from build123d import *

# Parameters (mm, degrees)
CROQUIS4_R              = 11
SALIENTE_EXTRUIR2_DEPTH = 25
CROQUIS5_R              = 3
SALIENTE_EXTRUIR3_DEPTH = 1.5
CROQUIS6_R              = 1.5
SALIENTE_EXTRUIR4_DEPTH = 0.5
CROQUIS7_R              = 1
SALIENTE_EXTRUIR5_DEPTH = 6
REDONDEO1_R             = 1
CROQUIS10_R             = 9.905946753
SALIENTE_EXTRUIR6_DEPTH = 1
CORTAR_EXTRUIR1_START   = 1
CROQUIS8_R              = 1.25
CORTAR_EXTRUIR1_DEPTH   = 6


with BuildPart() as part:
    # Croquis4 → Saliente-Extruir2 (new body)
    with BuildSketch(Plane(origin=(0, 0, 0), x_dir=(0, 0, -1), z_dir=(1, 0, 0))):
        Circle(CROQUIS4_R)
    extrude(amount=SALIENTE_EXTRUIR2_DEPTH)

    # Croquis5 → Saliente-Extruir3 (add)
    with BuildSketch(Plane(origin=(25, 0, 0), x_dir=(0, 0, -1), z_dir=(1, 0, 0))):
        Circle(CROQUIS5_R)
    extrude(amount=SALIENTE_EXTRUIR3_DEPTH)

    # Croquis6 → Saliente-Extruir4 (add)
    with BuildSketch(Plane(origin=(26.5, 0, 0), x_dir=(0, 0, -1), z_dir=(1, 0, 0))):
        Circle(CROQUIS6_R)
    extrude(amount=SALIENTE_EXTRUIR4_DEPTH)

    # Croquis7 → Saliente-Extruir5 (add)
    with BuildSketch(Plane(origin=(27, 0, 0), x_dir=(0, 0, -1), z_dir=(1, 0, 0))):
        Circle(CROQUIS7_R)
    extrude(amount=SALIENTE_EXTRUIR5_DEPTH)

    # Redondeo1
    redondeo1_edges = [part.edges().sort_by_distance(p)[0] for p in [
        (33, 0, 1),
    ]]
    fillet(redondeo1_edges, radius=REDONDEO1_R)

    # Croquis10 → Saliente-Extruir6 (add)
    with BuildSketch(Plane(origin=(25, 0, 0), x_dir=(0, 0, -1), z_dir=(1, 0, 0))):
        Circle(CROQUIS10_R)
    extrude(amount=SALIENTE_EXTRUIR6_DEPTH)

    # Croquis9 → Cortar-Revolución2 (revolve, cut)
    with BuildSketch(Plane.XY, mode=Mode.PRIVATE) as cortar_revoluci_n2_sk:
        Polygon((3.71935431, 11), (0, 11), (0, 10), (2.798724642, 10), align=None)
    revolve(cortar_revoluci_n2_sk.sketch.rotate(Axis((0, 0, 0), (1, 0, 0)), 90), axis=Axis((0, 0, 0), (1, 0, 0)), mode=Mode.SUBTRACT)

    # Croquis8 → Cortar-Extruir1 (cut)
    with BuildSketch(Plane(origin=(25, 0, 0), x_dir=(0, 0, -1), z_dir=(1, 0, 0)).offset(CORTAR_EXTRUIR1_START)):
        with Locations((0, 6)):
            Circle(CROQUIS8_R)
        with Locations((5.196152423, 3)):
            Circle(CROQUIS8_R)
        with Locations((5.196152423, -3)):
            Circle(CROQUIS8_R)
        with Locations((0, -6)):
            Circle(CROQUIS8_R)
        with Locations((-5.196152423, -3)):
            Circle(CROQUIS8_R)
        with Locations((-5.196152423, 3)):
            Circle(CROQUIS8_R)
    extrude(amount=-CORTAR_EXTRUIR1_DEPTH, mode=Mode.SUBTRACT)


solid = part.part
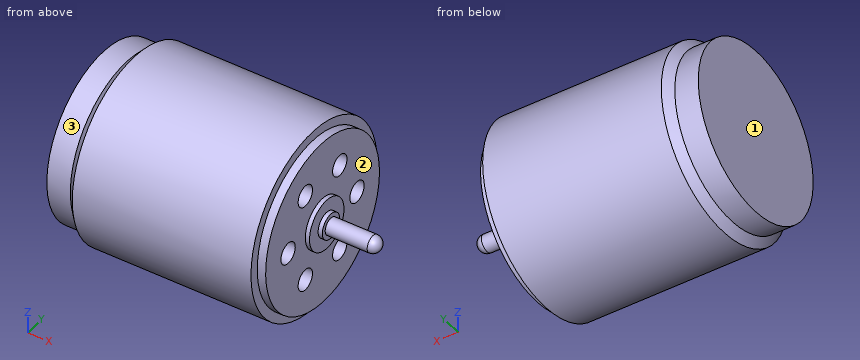
Verification items for the finished model (mm, model axes). Face numbers are marked on the shaded views. A direction names the side the tool comes from. Coordinates: 2 decimals unless noted, no trailing zeros. Write each loop counter-clockwise with the first axis right and the second up, starting at its lowest first coordinate (ties: lowest second). Pieces come first, ordered by that corner, then holes. Notation, with made-up numbers: M 88.25,26.5 L 101.25,26.5 A11 cw 101.25,44.5 Z; hole C 37,-17.75 d6. An arc over 180 degrees is marked long. Use a Markdown table: item, result.
Q1. Set-up check for the marked faces 1, 2 and 3: record each of +Z, -Z, +X, -X, +Y, -Y from which the full face is reachable in a straight line by a thin tool's end or side.
Reply:
| item | result |
|---|---|
| face 1 | +Z, -Z, -X, +Y, -Y |
| face 2 | +X |
| face 3 | -X |
Q2. Go/stop test with flat-tipped pins: P1, Ø12, axis at y = -4.5, z = -3, coming from the -X side; P2, Ø8, axis at y = 1, z = -8, coming from the +X side; P3, Ø1.2, axis at y = 3, z = 5.5, coming from the +X side; P4, Ø10, axis at x = 18.5, z = -6.5, coming from the +Y side. Record where each tip stops, or that it passes through.
Reply:
| item | result |
|---|---|
| P1 | stops at x = 0 |
| P2 | stops at x = 26 |
| P3 | stops at x = 20 |
| P4 | stops at y = 10.9 |
Q3. Sectioned sample at C-C, the plane x = 4.5. Record the boundary of the cut face in (y, z).
Reply:
| item | result |
|---|---|
| outline | C 0,0 d22 |
Q4. Thickness scan on line 1 (Y direction, x = 22.4, z = 0); line 2 (X direction, y = -5.75, z = 6.5); line 3 (X direction, y = -6.25, z = 0.25). Record the ranges inside material, lowest first.
Reply:
| item | result |
|---|---|
| line 1 | y = -11 to -7.25, -4.75 to 4.75, 7.25 to 11 |
| line 2 | x = 0 to 26 |
| line 3 | x = 0 to 20 |
Q5. Sectioned sample at B-B, the plane x = 27.5. Record the boundary of the cut face in (y, z), plus the area to 3 significant figures.
Reply:
| item | result |
|---|---|
| outline | C 0,0 d2 |
| area | 3.14 mm² |
